```python
from build123d import *

# Parameters (mm, degrees)
F0_R     = 10.16
F1_DEPTH = 11.43
F2_R     = 2.921
F3_DEPTH = 25.4
F5_DEPTH = 25.4
F7_DEPTH = 25.4


with BuildPart() as f1:
    # F0 (on Top) → F1 (new body)
    with BuildSketch(Plane.XY):
        Circle(F0_R)
    extrude(amount=F1_DEPTH)

    # F2 (on face) → F3 (cut)
    with BuildSketch(Plane.XY.offset(11.43)):
        Circle(F2_R)
    extrude(amount=-F3_DEPTH, mode=Mode.SUBTRACT)

    # F4 (on face) → F5 (cut)
    with BuildSketch(Plane.XY.offset(11.43)):
        with BuildLine():
            Line((-0.600534, -9.124259), (-0.600534, -4.044259))
            ThreePointArc((-0.600534, -4.044259), (-3.151262, -2.859133), (-4.061856, -0.198015))
            Line((-4.061856, -0.198015), (-9.141856, -0.198015))
            ThreePointArc((-9.141856, -0.198015), (-6.606663, -6.321767), (-0.600534, -9.124259))
        make_face()
    extrude(amount=-F5_DEPTH, mode=Mode.SUBTRACT)

    # F6 (on face) → F7 (cut)
    with BuildSketch(Plane.XY.offset(11.43)):
        with BuildLine():
            ThreePointArc((3.891585, -1.767314), (2.542541, -3.334315), (0.600534, -4.044259))
            Line((0.600534, -4.044259), (0.600534, -9.124259))
            ThreePointArc((0.600534, -9.124259), (5.960667, -6.782305), (8.971585, -1.767314))
            Line((8.971585, -1.767314), (3.891585, -1.767314))
        make_face()
        with BuildLine():
            ThreePointArc((0.874891, 4.022049), (3.387925, 2.803616), (4.06352, 0.093727))
            Line((4.06352, 0.093727), (9.14352, 0.093727))
            ThreePointArc((9.14352, 0.093727), (6.432661, 5.904461), (0.874891, 9.102049))
            Line((0.874891, 9.102049), (0.874891, 4.022049))
        make_face()
        with BuildLine():
            ThreePointArc((-4.046591, 0.563985), (-3.387877, 2.800717), (-1.365609, 3.961452))
            Line((-1.365609, 3.961452), (-1.365609, 9.041452))
            ThreePointArc((-1.365609, 9.041452), (-6.7496, 6.179148), (-9.126591, 0.563985))
            Line((-9.126591, 0.563985), (-4.046591, 0.563985))
        make_face()
    extrude(amount=-F7_DEPTH, mode=Mode.SUBTRACT)


solid = f1.part
```
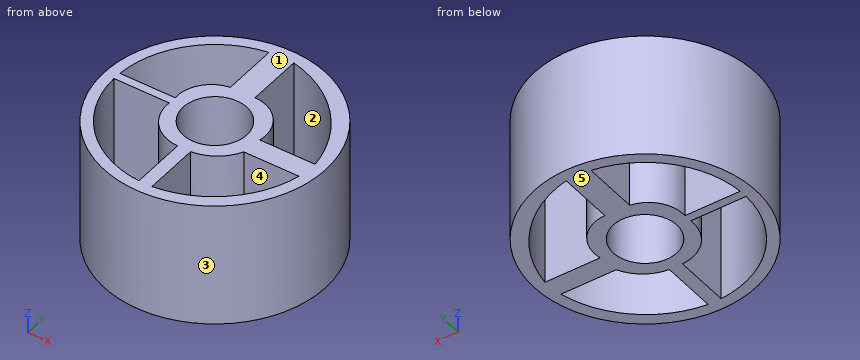
For this review, take the finished solid that the model builds, in its own axes (mm). Face numbers are marked on the shaded views. A direction names the side the tool comes from. Coordinates: 2 decimals unless noted, no trailing zeros. Write each loop counter-clockwise with the first axis right and the second up, starting at its lowest first coordinate (ties: lowest second). Pieces come first, ordered by that corner, then holes.
(1) Add section A-A on z = 8.5. Give the boundary of the cut face in (x, y).
(2) Add section D-D on x = 5. Give the boundary of the cut face in (y, z).
(3) Add section C-C on y = 7.25. Give the boundary of the cut face in (x, z).
(4) Add section B-B on x = 0. Give the boundary of the cut face in (y, z).
(5) Tool access review of the marked faces 1 and 2: name each direction out of +Z, -Z, +X, -X, +Y, -Y from which nothing blocks a thin tool from reaching the whole face with its end or side.
(6) For pin 1 Ø4 at (x, z) = (7, 4) entering from +Y; pin 2 Ø5.5 at (y, z) = (-6, 4.5) entering from +X; pin 3 Ø1.5 at (x, z) = (-4, 1) entering from -Y, all flat-tipped, find the tip position at first contact; note any pin that passes through.
(7) Wall thickness on probe 1 along Y at (x, z) = (0, 3); probe 2 along Y at (x, z) = (6.25, 8); probe 3 along X at (y, z) = (-4.25, 6): over which ranges is each line inside the solid? List them lowest first.
(8) The part is to be moulded in two halves that separate along Y. For the marked faces 3, 4 and 5, say which applies: +Y half, -Y half, draft (parallel to the pull), parting line (faces both ways), or undercut.
Answer sheet:
1. outline: circle Ø20.32 at (0, 0); hole (-9.14, -0.2) arc R9.14 ccw to (-0.6, -9.12) - (-0.6, -4.04) arc R3.59 cw to (-4.06, -0.2) - close; hole (-9.13, 0.56) - (-4.05, 0.56) arc R3.13 cw to (-1.37, 3.96) - (-1.37, 9.04) arc R9.12 ccw to start; hole circle Ø5.84 at (0, 0); hole (0.6, -9.12) arc R9.61 ccw to (8.97, -1.77) - (3.89, -1.77) arc R4.1 cw to (0.6, -4.04) - close; hole (0.87, 4.02) arc R3.3 cw to (4.06, 0.09) - (9.14, 0.09) arc R10.64 ccw to (0.87, 9.1) - close
2. outline: (-8.84, 0) - (-7.52, 0) - (-7.52, 11.43) - (-8.84, 11.43) - close; (-1.77, 0) - (0.09, 0) - (0.09, 11.43) - (-1.77, 11.43) - close; (7.21, 0) - (8.84, 0) - (8.84, 11.43) - (7.21, 11.43) - close
3. outline: (-7.12, 0) - (-5.58, 0) - (-5.58, 11.43) - (-7.12, 11.43) - close; (-1.37, 0) - (0.87, 0) - (0.87, 11.43) - (-1.37, 11.43) - close; (4.94, 0) - (7.12, 0) - (7.12, 11.43) - (4.94, 11.43) - close
4. outline: (-10.16, 0) - (-2.92, 0) - (-2.92, 11.43) - (-10.16, 11.43) - close; (2.92, 0) - (10.16, 0) - (10.16, 11.43) - (2.92, 11.43) - close
5. face 1: +Z, +X, -X, +Y, -Y
5. face 2: +Z, -Z
6. pin 1: stops at y = 8.84
6. pin 2: stops at x = 9.63
6. pin 3: stops at y = -9.63
7. probe 1: y = -10.16 to -2.92, 2.92 to 10.16
7. probe 2: y = -8.01 to -6.52, -1.77 to 0.09, 6.1 to 8.01
7. probe 3: x = -9.23 to -8.1, -0.6 to 0.6, 8.01 to 9.23
8. face 3: parting line
8. face 4: undercut
8. face 5: draft
